Design review of the part built by this model. Coordinates are the model's own, in mm. A direction names the side the tool comes from. Round coordinates to 2 decimals unless told otherwise and drop trailing zeros. Loops run counter-clockwise (first coordinate to the right, second up) from the corner with the lowest first, then second, coordinate; pieces in that order, holes last. Notation, with made-up numbers: M 47,35.25 L 102,35.25 A23 ccw 102,58.25 Z; hole C 73,70 d6. An arc over 180 degrees is marked long. Answer as CSV lines item,"result". Start each with the question number.
Autodesk Inventor part; units mm, degrees
ref_plane "YZ Plane" through (0, 0, 0) normal (1, 0, 0) x (0, 1, 0)
ref_plane "XZ Plane" through (0, 0, 0) normal (0, 1, 0) x (-1, 0, 0)
ref_plane "XY Plane" through (0, 0, 0) normal (0, 0, 1) x (1, 0, 0)
sketch "Base" plane through (0, 0, 0) normal (0, 0, 1) x (1, 0, 0)
  line L0 (-15.8, -12.35) -> (15.8, -12.35)
  line L1 (15.8, -12.35) -> (15.8, 12.35)
  line L2 (15.8, 12.35) -> (-15.8, 12.35)
  line L3 (-15.8, 12.35) -> (-15.8, -12.35)
  line L4 (-15.8, -12.35) -> (15.8, 12.35) construction
  line L5 (15.8, -12.35) -> (-15.8, 12.35) construction
  point P0 (0, 0)
  dimension "d0" = 31.6
  dimension "d1" = 24.7
extrude "BaseFeature" add sketch "Base" along normal blind 2
sketch "Switch" plane through (0, 0, 2) normal (0, 0, 1) x (1, 0, 0)
  line L0 (-12, -9) -> (12, -9)
  line L1 (12, -9) -> (12, 9)
  line L2 (12, 9) -> (-12, 9)
  line L3 (-12, 9) -> (-12, -9)
  line L4 (-12, -9) -> (12, 9) construction
  line L5 (12, -9) -> (-12, 9) construction
  point P0 (0, 0)
  dimension "d4" = 24
  dimension "d7" = 18
extrude "SwitchFeature" add sketch "Switch" along normal blind 6.5
sketch "SwitchProfile" plane through (-12, -9, 2) normal (0, -1, 0) x (1, 0, 0)
  line L0 (27.8, 0) -> (-3.8, 0)
  line L1 (24, 6.5) -> (0, 6.5)
  arc A0 (23, 0) -> (18, 6.5) centre (5.3894, -8.3735) ccw
  arc A1 (2.5453, 0.2566) -> (18, 6.5) centre (-6.2914, 44.3804) ccw
  arc A2 (2.5453, 0.2566) -> (1.5, 0) centre (5, -12) ccw
  line L2 (24, 0) -> (24, 6.5)
  line L3 (0, 0) -> (0, 6.5)
  point P0 (12, -2)
  point P1 (0, 3.25)
  dimension "d8" = 6
  dimension "d10" = 45
  dimension "d11" = 19.5
  dimension "d13" = 12.5
  dimension "d14" = 1
  dimension "d15" = 12
  dimension "d16" = 19
extrude "SwitchProfileFeature" cut sketch "SwitchProfile" against normal through all contours L0 A0 L1 L2 | L0 L3 L1 A1 A2
sketch "Body" plane through (0, 0, 0) normal (0, 0, -1) x (-1, 0, 0)
  line L0 (-15.35, -10.795) -> (15.35, -10.795)
  line L1 (15.35, -10.795) -> (15.35, 10.795)
  line L2 (15.35, 10.795) -> (-15.35, 10.795)
  line L3 (-15.35, 10.795) -> (-15.35, -10.795)
  line L4 (-15.35, -10.795) -> (15.35, 10.795) construction
  line L5 (15.35, -10.795) -> (-15.35, 10.795) construction
  line L6 (15.8, -12.35) -> (-15.8, -12.35)
  line L7 (15.8, 12.35) -> (15.8, -12.35)
  point P0 (0, 0)
  dimension "d19" = 21.59
  dimension "d20" = 1.555
  dimension "d29" = 30.7
extrude "BodyFeature" add sketch "Body" along normal blind 17
sketch "Pins" plane through (0, 0, -17) normal (0, 0, -1) x (-1, 0, 0)
  line L0 (11.5, -6.6456) -> (-11.5, -6.6456)
  line L1 (-11.5, -6.6456) -> (-11.5, 6.6456)
  line L2 (-11.5, 6.6456) -> (11.5, 6.6456)
  line L3 (11.5, 6.6456) -> (11.5, -6.6456)
  line L4 (11.5, -6.6456) -> (-11.5, 6.6456) construction
  line L5 (-11.5, -6.6456) -> (11.5, 6.6456) construction
  line L6 (-15.35, -10.795) -> (15.35, -10.795)
  point P0 (0, 0)
  point P1 (0, -10.795)
  dimension "d25" = 23
extrude "PinsFeature" add sketch "Pins" along normal blind 10.5
properties part number "IlluminatedSwitch12V10A"
Item 1: Consider section C-C, the plane z = -16.5. Write out the cut boundary in (x, y) (3 decimals).
Item 2: Consider section B-B, the plane y = -2.5. Write out the cut boundary in (x, z), then the cut area to 3 significant figures.
Item 3: To check wall thickness, follow line 1 (Z direction, x = 13, y = 10); line 2 (X direction, y = 3.25, z = -16.5); line 3 (Y direction, x = -8, z = -22.5). State the ranges of each line that lie inside material, in increasing order.
Item 4: Consider section D-D, the plane x = -4. Write out the cut boundary in (y, z) (3 decimals).
Item 5: Insertion check: pin 1 Ø1.5 at (x, z) = (-4, -1) entering from +Y (3 decimals); pin 2 Ø5 at (y, z) = (-0.5, -24.5) entering from -X; pin 3 Ø5 at (x, z) = (-4.5, 6) entering from -Y. Each pin has a flat end and moves straight along its axis. Give the tip position at first contact, or say it passes through.
Item 6: Consider section A-A, the plane x = 13.5. Write out the cut boundary in (y, z) (3 decimals).
Item 7: Tool access review of faces 1 (the face through (15.35, 0, -8)), 2 (the face through (2, -9, 4)), 3 (the face through (0, -10.795, -8)): name each direction out of +Z, -Z, +X, -X, +Y, -Y from which nothing blocks a thin tool from reaching the whole face with its end or side.
Found:
1,outline,"M -15.35,-10.795 L 15.35,-10.795 L 15.35,10.795 L -15.35,10.795 Z"
2,outline,"M -15.8,0 L -15.35,0 L -15.35,-17 L -11.5,-17 L -11.5,-27.5 L 11.5,-27.5 L 11.5,-17 L 15.35,-17 L 15.35,0 L 15.8,0 L 15.8,2 L 11,2 A19.5 ccw 6,8.5 A45 cw -9.45,2.26 A12.5 ccw -10.5,2 L -15.8,2 Z"
2,area,"889 mm^2"
3,line 1,"z = -17 to 2"
3,line 2,"x = -15.35 to 15.35"
3,line 3,"y = -6.65 to 6.65"
4,outline,"M -12.35,0 L -10.795,0 L -10.795,-17 L -6.646,-17 L -6.646,-27.5 L 6.646,-27.5 L 6.646,-17 L 10.795,-17 L 10.795,0 L 12.35,0 L 12.35,2 L 9,2 L 9,3.71 L -9,3.71 L -9,2 L -12.35,2 Z"
5,pin 1,"stops at y = 10.795"
5,pin 2,"stops at x = -11.5"
5,pin 3,"stops at y = -9"
6,outline,"M -12.35,0 L -10.795,0 L -10.795,-17 L 10.795,-17 L 10.795,0 L 12.35,0 L 12.35,2 L -12.35,2 Z"
7,face 1,"-Z, +X, +Y, -Y"
7,face 2,"+Z, +X, -X, -Y"
7,face 3,"-Z, +X, -X, -Y"
